```python
from build123d import *

# Parameters (mm, degrees)
F2_W            = 0.2
F2_H            = 0.22
F3_ANGLE        = 20
F3_COPIES_COUNT = 12
F5_DEPTH        = 0.15


# Not quite as in the source:
# - a pattern or mirror of a feature is missing from the dataset's text; its kind, count and spacing are read off the source's solid


with BuildPart() as f1:
    # F0 (on Front) → F1 (revolve)
    with BuildSketch(Plane.XZ):
        with BuildLine():
            Line((1, 0.85), (0.87, 0.85))
            ThreePointArc((0.87, 0.85), (0.8134314575, 0.8734314575), (0.79, 0.93))
            Line((0.79, 0.93), (0.79, 1.11))
            ThreePointArc((0.79, 1.11), (0.8134314575, 1.1665685425), (0.87, 1.19))
            Line((0.87, 1.19), (1.1, 1.19))
            Line((1.1, 1.19), (1.1, 1.54))
            Line((1.1, 1.54), (1.2, 1.54))
            Line((1.2, 1.54), (1.2, 1.64))
            Line((1.2, 1.64), (1.12, 1.64))
            Line((1.12, 1.64), (1.0590550792, 1.64))
            add(Edge.make_bspline(
                [(1.0590550792, 1.64), (1.25, 2.3421209771), (1.2635455001, 2.685534462), (1.2259744013, 3.2558219262), (0.9930693577, 3.4693235058), (0.91, 3.5233867214)],
                knots=[0, 0, 0, 0, 0.3714125336, 0.6273384476, 0.7316891336, 0.7316891336, 0.7316891336, 0.7316891336], degree=3))
            Line((0.91, 3.5233867214), (0.91, 3.3833867214))
            Line((0.91, 3.3833867214), (0.77, 3.4602341654))
            Line((0.77, 3.4602341654), (0.77, 3.6002341654))
            add(Edge.make_bspline(
                [(0.77, 3.6002341654), (0.6784642229, 3.6425426702), (0.5744947558, 3.6771881754), (0.46, 3.7024604996)],
                knots=[0.7852748547, 0.7852748547, 0.7852748547, 0.7852748547, 0.8822719118, 0.8822719118, 0.8822719118, 0.8822719118], degree=3))
            Line((0.46, 3.7024604996), (0.46, 3.5624604996))
            Line((0.46, 3.5624604996), (0.32, 3.5878456739))
            Line((0.32, 3.5878456739), (0.32, 3.7278456739))
            add(Edge.make_bspline(
                [(0.32, 3.7278456739), (0.2195553432, 3.7423008552), (0.1125378698, 3.75), (0, 3.75)],
                knots=[0.9204576606, 0.9204576606, 0.9204576606, 0.9204576606, 1, 1, 1, 1], degree=3))
            Line((0, 3.75), (0, 2.75))
            Line((0, 2.75), (0, 2.5))
            Line((0, 2.5), (-0.35, 2.5))
            Line((-0.35, 2.5), (-0.35, 2.2))
            Line((-0.35, 2.2), (0.02, 2.2))
            Line((0.02, 2.2), (0.02, 2.15))
            Line((0.02, 2.15), (0.02, 0))
            Line((0.02, 0), (0.5, 0))
            Line((0.5, 0), (0.5, 0.515))
            Line((0.5, 0.515), (1, 0.515))
            Line((1, 0.515), (1, 0.85))
        make_face()
    revolve(axis=Axis((1.052, 0, 0), (1, 0, 0)))

    # F2 (on Front) → F3 (revolve, cut)
    with BuildSketch(Plane.XZ):
        with Locations((1.07, 1.4)):
            Rectangle(F2_W, F2_H)
    f3 = revolve(axis=Axis((1.36, 0, 0), (-1, 0, 0)), revolution_arc=F3_ANGLE, mode=Mode.SUBTRACT)

    # F3_copies: F3 ×12 about axis
    f3_copies_axis = Axis((0, 0, 0), (1, 0, 0))
    for i in range(1, F3_COPIES_COUNT):
        add(f3.rotate(f3_copies_axis, i * 360 / F3_COPIES_COUNT), mode=Mode.SUBTRACT)

    # F4 (on face) → F5 (join)
    with BuildSketch(Plane.YZ.offset(0.79)):
        with BuildLine():
            Line((-0.3895609432, 1.0703098951), (-0.2696546218, 0.7408699845))
            ThreePointArc((-0.2696546218, 0.7408699845), (-0.0687151015, 0.7854172037), (0.1369072395, 0.7764395384))
            Line((0.1369072395, 0.7764395384), (0.1977852744, 1.1216960307))
            ThreePointArc((0.1977852744, 1.1216960307), (-0.099270391, 1.1346657611), (-0.3895609432, 1.0703098951))
        make_face()
        with BuildLine():
            Line((-1.1216960307, 0.1977852744), (-0.7764395384, 0.1369072395))
            ThreePointArc((-0.7764395384, 0.1369072395), (-0.7145488017, 0.3331995784), (-0.603962745, 0.5067849166))
            Line((-0.603962745, 0.5067849166), (-0.8725246207, 0.7321350874))
            ThreePointArc((-0.8725246207, 0.7321350874), (-1.0322845694, 0.4813622001), (-1.1216960307, 0.1977852744))
        make_face()
        with BuildLine():
            Line((-0.7321350874, -0.8725246207), (-0.5067849166, -0.603962745))
            ThreePointArc((-0.5067849166, -0.603962745), (-0.6458337002, -0.4522176253), (-0.7408699845, -0.2696546218))
            Line((-0.7408699845, -0.2696546218), (-1.0703098951, -0.3895609432))
            ThreePointArc((-1.0703098951, -0.3895609432), (-0.9330141784, -0.653303561), (-0.7321350874, -0.8725246207))
        make_face()
        with BuildLine():
            Line((0.3895609432, -1.0703098951), (0.2696546218, -0.7408699845))
            ThreePointArc((0.2696546218, -0.7408699845), (0.0687151015, -0.7854172037), (-0.1369072395, -0.7764395384))
            Line((-0.1369072395, -0.7764395384), (-0.1977852744, -1.1216960307))
            ThreePointArc((-0.1977852744, -1.1216960307), (0.099270391, -1.1346657611), (0.3895609432, -1.0703098951))
        make_face()
        with BuildLine():
            Line((1.1216960307, -0.1977852744), (0.7764395384, -0.1369072395))
            ThreePointArc((0.7764395384, -0.1369072395), (0.7145488017, -0.3331995784), (0.603962745, -0.5067849166))
            Line((0.603962745, -0.5067849166), (0.8725246207, -0.7321350874))
            ThreePointArc((0.8725246207, -0.7321350874), (1.0322845694, -0.4813622001), (1.1216960307, -0.1977852744))
        make_face()
        with BuildLine():
            Line((0.7321350874, 0.8725246207), (0.5067849166, 0.603962745))
            ThreePointArc((0.5067849166, 0.603962745), (0.6458337002, 0.4522176253), (0.7408699845, 0.2696546218))
            Line((0.7408699845, 0.2696546218), (1.0703098951, 0.3895609432))
            ThreePointArc((1.0703098951, 0.3895609432), (0.9330141784, 0.653303561), (0.7321350874, 0.8725246207))
        make_face()
    extrude(amount=F5_DEPTH)


solid = f1.part
```
CAD build for the part. Positions are in the model's coordinates, mm. Round coordinates to 2 decimals unless told otherwise and drop trailing zeros. Answer in a Markdown table with one row per item. Add a question column.
(1) Mould opens along Z. For faces 1 (the face through (0, -3, 0)), 2 (the face through (-0.18, 2.44, -0.54)), 3 (the face through (0.5, 0, 0)) say: +Z half, -Z half, draft (parallel to the pull), parting line (faces both ways), or undercut.
(2) Probe L1, parallel to Y at x = -0.1, z = 0; L2, parallel to Y at x = 0.95, z = 0 (3 decimals). List the from-to ranges inside material, lowest first. Write a range as [from, to].
(3) Drop flat-ended pins along their axis: pin 1 Ø1.4 at (y, z) = (0, 0) entering from +X; pin 2 Ø0.5 at (y, z) = (1, -1) entering from +X; pin 3 Ø0.5 at (y, z) = (-1, 0.5) entering from +X. Give the stop position or say it passes through.
Data:
| question | item | result |
|---|---|---|
| 1 | face 1 | draft |
| 1 | face 2 | parting line |
| 1 | face 3 | undercut |
| 2 | L1 | y = [-2.5, -2.2], [2.2, 2.5] |
| 2 | L2 | y = [-3.496, -1.19], [-0.85, -0.515], [0.515, 0.85], [1.19, 3.496] |
| 3 | pin 1 | stops at x = 1 |
| 3 | pin 2 | stops at x = 1.2 |
| 3 | pin 3 | stops at x = 1.1 |
